Answer from the drawing. Dimensions are ordinates in mm from the lowest x, y and z of the part. Give positions to 0.01 mm unless a question says otherwise; leave off trailing zeros. Order: outer loops, then holes, each group sorted by start corner. A loop starts at its lowest first (then second) coordinate and runs counter-clockwise, first axis right, second up.
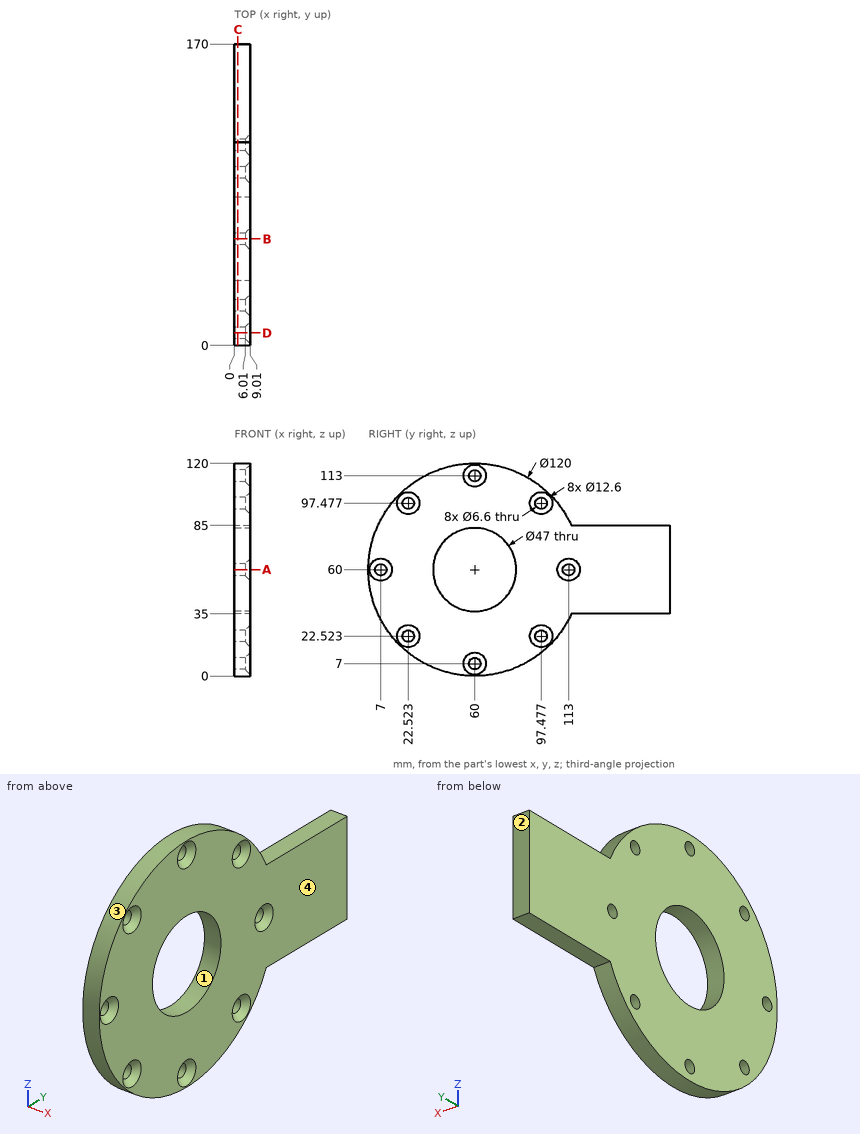
1. The mould has two halves that part along Y. Classify the marked faces 1, 2, 3 and 4: pulls with the +Y half, pulls with the -Y half, needs draft (parallel to the pull), parting line crosses it, or undercut.
Findings below:
face 1: undercut
face 2: pulls with the +Y half
face 3: parting line crosses it
face 4: needs draft
2. The part is cut by section D-D (y = 7). Write down the section's boundary in (x, z) (1 decimal).
Findings below:
outline: (0, 31.9) - (9, 31.9) - (9, 53.7) - (6, 56.7) - (0, 56.7) - close; (0, 63.3) - (6, 63.3) - (9, 66.3) - (9, 88.1) - (0, 88.1) - close
3. The part is cut by section B-B (y = 60). Write down the section's boundary in (x, z), then the cut area to 3 significant figures.
Findings below:
outline: (0, 0) - (9.01, 0) - (9.01, 0.7) - (6.01, 3.7) - (0, 3.7) - close; (0, 10.3) - (6.01, 10.3) - (9.01, 13.3) - (9.01, 36.5) - (0, 36.5) - close; (0, 83.5) - (9.01, 83.5) - (9.01, 106.7) - (6.01, 109.7) - (0, 109.7) - close; (0, 116.3) - (6.01, 116.3) - (9.01, 119.3) - (9.01, 120) - (0, 120) - close
area: 521 mm2
4. Given P1, Ø8.5, axis at y = 60, z = 113, coming from the +X side; P2, Ø2, axis at x = 4, z = 50, coming from the -Y side; P3, Ø6, axis at y = 97.48, z = 97.48, coming from the -X side; P4, Ø2, axis at x = 7, z = 50.5, coming from the -Y side (1 decimal), each flat-ended and moving along its own axis, determine where each tip first touches the part or whether it passes through.
Findings below:
P1: stops at x = 6.96
P2: stops at y = 0.68
P3: passes through
P4: stops at y = 0.6
5. Straight lines are drawn through the part: probe 1 along Y at (x, z) = (2.5, 62) (1 decimal); probe 2 along Z at (x, y) = (3.5, 96.5) (1 decimal); probe 3 along Z at (x, y) = (4.25, 156). For each, find the intervals that lie inside material, in ascending order.
Findings below:
probe 1: y = 0 to 4.4, 9.6 to 36.6, 83.4 to 110.4, 115.6 to 170
probe 2: z = 12.4 to 19.4, 25.7 to 94.3, 100.6 to 107.6
probe 3: z = 35 to 85
6. The part is cut by section A-A (z = 60). Write down the section's boundary in (x, y), then the cut area to 3 significant figures.
Findings below:
outline: (0, 0) - (9.01, 0) - (9.01, 0.7) - (6.01, 3.7) - (0, 3.7) - close; (0, 10.3) - (6.01, 10.3) - (9.01, 13.3) - (9.01, 36.5) - (0, 36.5) - close; (0, 83.5) - (9.01, 83.5) - (9.01, 106.7) - (6.01, 109.7) - (0, 109.7) - close; (0, 116.3) - (6.01, 116.3) - (9.01, 119.3) - (9.01, 170) - (0, 170) - close
area: 971 mm2
7. The part is cut by section C-C (x = 2). State how many separate pieces and enclosed holes the cut face has, then the cut area to 3 significant figures.
Findings below:
separate pieces: 1
enclosed holes: 9
area: 11,900 mm2
